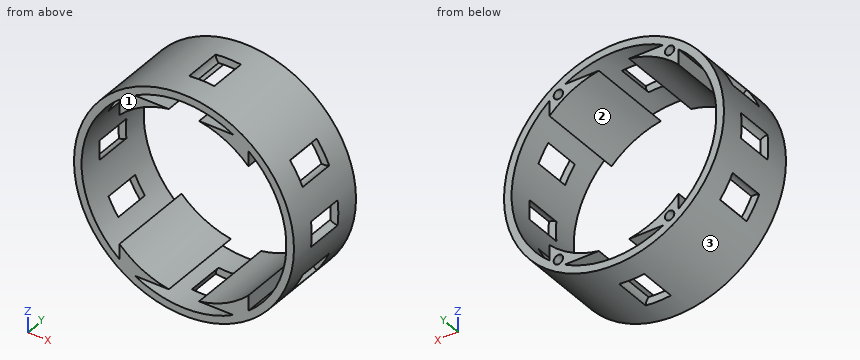
```python
from build123d import *

# Parameters (mm, degrees)
SKETCH1_R               = 43.5
SKETCH1_R_2             = 40.5
BOSS_EXTRUDE1_DEPTH     = 35
SKETCH2_R               = 1.85
CUT_EXTRUDE1_DEPTH      = 15
CUT_EXTRUDE3_DEPTH      = 7.5
CUT_EXTRUDE3_DEPTH_BACK = 7.5


with BuildPart() as part:
    # Sketch1 → Boss-Extrude1 (new body)
    with BuildSketch(Plane(origin=(0, 0, 0), x_dir=(1, 0, 0), z_dir=(0, 1, 0))):
        Circle(SKETCH1_R)
        Circle(SKETCH1_R_2, mode=Mode.SUBTRACT)
        with BuildLine():
            Line((-25.5, -25.411611519), (-25.5, -31.464265445))
            ThreePointArc((-25.5, -31.464265445), (-22.587110133, -33.616550327), (-19.49358869, -35.5))
            Line((-19.49358869, -35.5), (-5.979130372, -35.5))
            ThreePointArc((-5.979130372, -35.5), (-16.528091474, -31.981591459), (-25.5, -25.411611519))
        make_face()
        with BuildLine():
            Line((5.979130372, -35.5), (19.49358869, -35.5))
            ThreePointArc((19.49358869, -35.5), (22.587110133, -33.616550327), (25.5, -31.464265445))
            Line((25.5, -31.464265445), (25.5, -25.411611519))
            ThreePointArc((25.5, -25.411611519), (16.528091474, -31.981591459), (5.979130372, -35.5))
        make_face()
        with BuildLine():
            ThreePointArc((25.5, 31.464265445), (22.587110133, 33.616550327), (19.49358869, 35.5))
            Line((19.49358869, 35.5), (5.979130372, 35.5))
            ThreePointArc((5.979130372, 35.5), (16.528091474, 31.981591459), (25.5, 25.411611519))
            Line((25.5, 25.411611519), (25.5, 31.464265445))
        make_face()
        with BuildLine():
            ThreePointArc((-19.49358869, 35.5), (-22.587110133, 33.616550327), (-25.5, 31.464265445))
            Line((-25.5, 31.464265445), (-25.5, 25.411611519))
            ThreePointArc((-25.5, 25.411611519), (-16.528091474, 31.981591459), (-5.979130372, 35.5))
            Line((-5.979130372, 35.5), (-19.49358869, 35.5))
        make_face()
    extrude(amount=BOSS_EXTRUDE1_DEPTH)

    # Sketch2 → Cut-Extrude1 (cut)
    with BuildSketch(Plane(origin=(0, 35, 0), x_dir=(1, 0, 0), z_dir=(0, 1, 0))):
        with Locations((-22, 32.606393643)):
            Circle(SKETCH2_R)
        with Locations((22, 32.5)):
            Circle(SKETCH2_R)
        with Locations((22, -32.5)):
            Circle(SKETCH2_R)
        with Locations((-22, -32.393606357)):
            Circle(SKETCH2_R)
    extrude(amount=-CUT_EXTRUDE1_DEPTH, mode=Mode.SUBTRACT)

    # Sketch6 → Cut-Extrude3 (cut, two sides)
    with BuildSketch(Plane(origin=(0, 17.5, 0), x_dir=(1, 0, 0), z_dir=(0, 1, 0))) as cut_extrude3_sk:
        with BuildLine():
            ThreePointArc((-40.316091954, 3.855221077), (-41.673709906, 4.654531608), (-43.212643678, 4.991735805))
            ThreePointArc((-43.212643678, 4.991735805), (-43.5, 0), (-43.212643678, -4.991735805))
            ThreePointArc((-43.212643678, -4.991735805), (-41.673709906, -4.654531608), (-40.316091954, -3.855221077))
            ThreePointArc((-40.316091954, -3.855221077), (-40.5, 0), (-40.316091954, 3.855221077))
        make_face()
        with BuildLine():
            ThreePointArc((-39.919115092, -17.283351823), (-37.672105065, -21.75), (-34.927379288, -25.929291855))
            ThreePointArc((-34.927379288, -25.929291855), (-33.763225644, -24.867797568), (-32.987149275, -23.496765367))
            ThreePointArc((-32.987149275, -23.496765367), (-35.074028853, -20.25), (-36.842370352, -16.819326587))
            ThreePointArc((-36.842370352, -16.819326587), (-38.417757252, -16.805912337), (-39.919115092, -17.283351823))
        make_face()
        with BuildLine():
            ThreePointArc((4.991735805, -43.212643678), (4.654531608, -41.673709906), (3.855221077, -40.316091954))
            ThreePointArc((3.855221077, -40.316091954), (0, -40.5), (-3.855221077, -40.316091954))
            ThreePointArc((-3.855221077, -40.316091954), (-4.654531608, -41.673709906), (-4.991735805, -43.212643678))
            ThreePointArc((-4.991735805, -43.212643678), (0, -43.5), (4.991735805, -43.212643678))
        make_face()
        with BuildLine():
            ThreePointArc((34.927379288, -25.929291855), (37.672105065, -21.75), (39.919115092, -17.283351823))
            ThreePointArc((39.919115092, -17.283351823), (38.417757252, -16.805912337), (36.842370352, -16.819326587))
            ThreePointArc((36.842370352, -16.819326587), (35.074028853, -20.25), (32.987149275, -23.496765367))
            ThreePointArc((32.987149275, -23.496765367), (33.763225644, -24.867797568), (34.927379288, -25.929291855))
        make_face()
        with BuildLine():
            ThreePointArc((40.316091954, -3.855221077), (40.5, 0), (40.316091954, 3.855221077))
            ThreePointArc((40.316091954, 3.855221077), (41.673709906, 4.654531608), (43.212643678, 4.991735805))
            ThreePointArc((43.212643678, 4.991735805), (43.5, 0), (43.212643678, -4.991735805))
            ThreePointArc((43.212643678, -4.991735805), (41.673709906, -4.654531608), (40.316091954, -3.855221077))
        make_face()
        with BuildLine():
            ThreePointArc((39.919115092, 17.283351823), (37.672105065, 21.75), (34.927379288, 25.929291855))
            ThreePointArc((34.927379288, 25.929291855), (33.763225644, 24.867797568), (32.987149275, 23.496765367))
            ThreePointArc((32.987149275, 23.496765367), (35.074028853, 20.25), (36.842370352, 16.819326587))
            ThreePointArc((36.842370352, 16.819326587), (38.417757252, 16.805912337), (39.919115092, 17.283351823))
        make_face()
        with BuildLine():
            ThreePointArc((3.855221077, 40.316091954), (0, 40.5), (-3.855221077, 40.316091954))
            ThreePointArc((-3.855221077, 40.316091954), (-4.654531608, 41.673709906), (-4.991735805, 43.212643678))
            ThreePointArc((-4.991735805, 43.212643678), (0, 43.5), (4.991735805, 43.212643678))
            ThreePointArc((4.991735805, 43.212643678), (4.654531608, 41.673709906), (3.855221077, 40.316091954))
        make_face()
        with BuildLine():
            ThreePointArc((-34.927379288, 25.929291855), (-37.672105065, 21.75), (-39.919115092, 17.283351823))
            ThreePointArc((-39.919115092, 17.283351823), (-38.417757252, 16.805912337), (-36.842370352, 16.819326587))
            ThreePointArc((-36.842370352, 16.819326587), (-35.074028853, 20.25), (-32.987149275, 23.496765367))
            ThreePointArc((-32.987149275, 23.496765367), (-33.763225644, 24.867797568), (-34.927379288, 25.929291855))
        make_face()
    extrude(amount=CUT_EXTRUDE3_DEPTH, mode=Mode.SUBTRACT)
    extrude(cut_extrude3_sk.sketch, amount=-CUT_EXTRUDE3_DEPTH_BACK, mode=Mode.SUBTRACT)


solid = part.part
```
The listing builds one solid part. Answer for the finished solid, in the listing's coordinates (mm). Face numbers are marked on the shaded views. Round coordinates to 2 decimals unless told otherwise and drop trailing zeros. Write each loop counter-clockwise with the first axis right and the second up, starting at its lowest first coordinate (ties: lowest second). Pieces come first, ordered by that corner, then holes. Notation, with made-up numbers: (87.5, 9.25) -> (134.5, 9.25) arc R13 ccw to (134.5, 21.25) -> close; hole circle Ø10 at (79, -27.75). An arc over 180 degrees is marked (long way). Use CSV: the item, a comma, the result in double quotes. Start each with the question number.
(1) Section A-A on x = 0 is taken. Give the vertices of the cut face in (y, z).
(2) The mould has two halves that part along X. Classify the marked faces 1, 2 and 3: released by +X, released by -X, zero draft, split by the parting line, or undercut.
(3) Section B-B on z = 0 is taken. Give the vertices of the cut face in (x, y).
(4) Consider L1, parallel to X at y = 6, z = -28; L2, parallel to Z at x = -16, y = 3.5; L3, parallel to Z at x = -0.5, y = 6. Determine where each line is inside the solid, lowest interval first. Write a range as from..to.
(5) Section D-D on y = 26.5 is taken. Give the vertices of the cut face in (x, z).
(6) Each of these flat-tipped pins is pushed along its axis until it touches: pin 1 (4 mm diameter, centred on x = 12, y = 28.5, fed in from +Z) (3 decimals); pin 2 (7 mm diameter, centred on x = -13.5, y = 24, fed in from -Z) (3 decimals); pin 3 (1.5 mm diameter, centred on y = 20.5, z = 21.5, fed in from +X); pin 4 (3 mm diameter, centred on y = 25.5, z = 29.5, fed in from +X). Where does it stop, or does it pass through?
(7) Section C-C on x = 22 is taken. Give the vertices of the cut face in (y, z).
A:
1,outline,"(0, -43.5) -> (10, -43.5) -> (10, -40.5) -> (0, -40.5) -> close; (0, 40.5) -> (10, 40.5) -> (10, 43.5) -> (0, 43.5) -> close; (25, -43.5) -> (35, -43.5) -> (35, -40.5) -> (25, -40.5) -> close; (25, 40.5) -> (35, 40.5) -> (35, 43.5) -> (25, 43.5) -> close"
2,face 1,"zero draft"
2,face 2,"undercut"
2,face 3,"split by the parting line"
3,outline,"(-43.5, 0) -> (-40.5, 0) -> (-40.5, 10) -> (-43.5, 10) -> close; (-43.5, 25) -> (-40.5, 25) -> (-40.5, 35) -> (-43.5, 35) -> close; (40.5, 0) -> (43.5, 0) -> (43.5, 10) -> (40.5, 10) -> close; (40.5, 25) -> (43.5, 25) -> (43.5, 35) -> (40.5, 35) -> close"
4,L1,"x = -33.29..-29.26, -25.5..-22.63, 22.63..25.5, 29.26..33.29"
4,L2,"z = -40.45..-37.21, -35.5..-32.25, 32.25..35.5, 37.21..40.45"
4,L3,"z = -43.5..-40.5, 40.5..43.5"
5,outline,"circle Ø87 at (0, 0); hole (-25.5, -31.46) -> (-25.5, -25.41) arc R36 ccw to (-5.98, -35.5) -> (-19.49, -35.5) arc R40.5 ccw to (19.49, -35.5) -> (5.98, -35.5) arc R36 ccw to (25.5, -25.41) -> (25.5, -31.46) arc R40.5 ccw to (25.5, 31.46) -> (25.5, 25.41) arc R36 ccw to (5.98, 35.5) -> (19.49, 35.5) arc R40.5 ccw to (-19.49, 35.5) -> (-5.98, 35.5) arc R36 ccw to (-25.5, 25.41) -> (-25.5, 31.46) arc R40.5 ccw to start; hole circle Ø3.7 at (-22, -32.61); hole circle Ø3.7 at (-22, 32.39); hole circle Ø3.7 at (22, -32.5); hole circle Ø3.7 at (22, 32.5)"
6,pin 1,"stops at z = 42.335"
6,pin 2,"stops at z = -42.335"
6,pin 3,"passes through"
6,pin 4,"stops at x = 33.29"
7,outline,"(0, -37.53) -> (35, -37.53) -> (35, -34.35) -> (20, -34.35) -> (20, -30.65) -> (35, -30.65) -> (35, -28.5) -> (0, -28.5) -> close; (0, 28.5) -> (35, 28.5) -> (35, 30.65) -> (20, 30.65) -> (20, 34.35) -> (35, 34.35) -> (35, 37.53) -> (0, 37.53) -> close"
